```python
from build123d import *

# Parameters (mm, degrees)
F1_DEPTH       = 12
F2_D           = 3.3
F2_CBORE_D     = 6.5
F2_CBORE_DEPTH = 3
F3_R           = 5


with BuildPart() as f1:
    # F0 (on Top) → F1 (new body)
    with BuildSketch(Plane.XY):
        with BuildLine():
            Line((40, 10), (0, 10))
            ThreePointArc((0, 10), (-10, 0), (0, -10))
            Line((0, -10), (40, -10))
            ThreePointArc((40, -10), (50, 0), (40, 10))
        make_face()
    extrude(amount=F1_DEPTH)

    # F2 (through all)
    with Locations(Plane(origin=(0, 0, 0), x_dir=(1, 0, 0), z_dir=(0, 0, -1))):
        with Locations((40, 0), (0, 0)):
            CounterBoreHole(F2_D / 2, F2_CBORE_D / 2, F2_CBORE_DEPTH)

    # F3
    f3_edges = [f1.edges().sort_by_distance(p)[0] for p in [
        (20, -10, 0),
    ]]
    fillet(f3_edges, radius=F3_R)


solid = f1.part
```
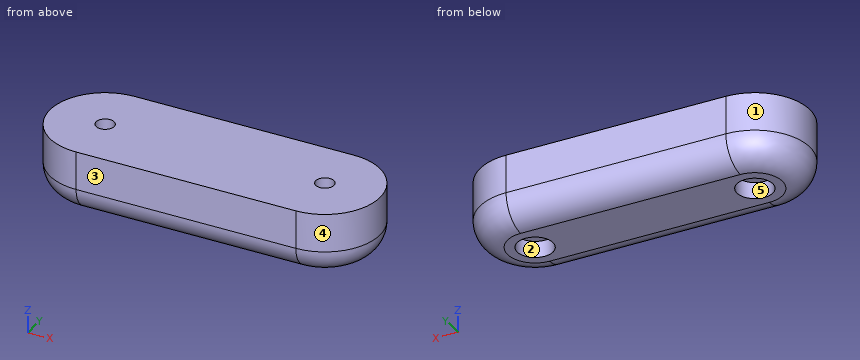
Geometry check sheet. Reference: the model listing, model coordinates, mm. Face numbers are marked on the shaded views. A direction names the side the tool comes from. Coordinates: 2 decimals unless noted, no trailing zeros. Order: outer loops, then holes, each group sorted by start corner. A loop starts at its lowest first (then second) coordinate and runs counter-clockwise, first axis right, second up. Notation, with made-up numbers: (84, 39.5) - (93, 39.5) arc R11 ccw to (93, 57.5) - close; hole circle Ø4 at (-26.75, 23). An arc over 180 degrees is marked (long way). Answer as a JSON object with one key per item and string values. Group by question number.
Item 1: Draft check along Y on the marked faces 3, 4 and 5. Enter one of: +Y half, -Y half, draft (parallel to the pull), parting line (faces both ways), or undercut.
Item 2: Depth check by flat-ended pin: pin 1 Ø3 at (x, y) = (40, 0.5) entering from -Z; pin 2 Ø1.5 at (y, z) = (4, 9) entering from +X. Enter the tip coordinate at first touch or a pass-through.
Item 3: Sectioned sample at C-C, the plane x = 11.5. Record the cut outline in (y, z).
Item 4: Sectioned sample at B-B, the plane y = 0. Give the number of separate pieces and of enclosed holes in the cut face, and give its area (3 significant figures).
Item 5: Sectioned sample at A-A, the plane z = 6. Record the cut outline in (x, y).
Item 6: Scan lines: probe 1 along Y at (x, z) = (0, 8.5); probe 2 along X at (y, z) = (-2.5, 2.75); probe 3 along X at (y, z) = (1, 3.25). Record each from-to range of solid material in increasing order.
Item 7: Tool access check on the marked faces 1 and 2. Record the directions out of +Z, -Z, +X, -X, +Y, -Y that give a thin tool (end or side, any length) a straight path to the whole face; none if there is none.
Resolved:
{
 "1": {"face 3": "-Y half", "face 4": "parting line", "face 5": "undercut"},
 "2": {"pin 1": "z = 3", "pin 2": "x = 49.46"},
 "3": {"outline": "(-10, 5) arc R5 ccw to (-5, 0) - (5, 0) arc R5 ccw to (10, 5) - (10, 12) - (-10, 12) - close"},
 "4": {"separate pieces": "3", "enclosed holes": "0", "area": "611 mm^2"},
 "5": {"outline": "(0, -10) - (40, -10) arc R10 ccw to (40, 10) - (0, 10) arc R10 ccw to start; hole circle Ø3.3 at (0, 0); hole circle Ø3.3 at (40, 0)"},
 "6": {"probe 1": "-10 to -1.65, 1.65 to 10", "probe 2": "-9.13 to -2.08, 2.08 to 37.92, 42.08 to 49.13", "probe 3": "-9.63 to -1.31, 1.31 to 38.69, 41.31 to 49.63"},
 "7": {"face 1": "+Z, -Z, -X", "face 2": "-Z"}
}
